from build123d import *

# Parameters (mm, degrees)
SKETCH1_R           = 12.5
BOSS_EXTRUDE1_DEPTH = 8
SKETCH2_R           = 10
BOSS_EXTRUDE2_DEPTH = 2
CUT_EXTRUDE1_REACH  = 22.31
SKETCH3_R           = 1.75
SKETCH4_R           = 3
CUT_EXTRUDE2_DEPTH  = 5
SKETCH5_R           = 9
SKETCH5_R_2         = 8
BOSS_EXTRUDE3_DEPTH = 1.5
CHAMFER1_SIZE       = 0.5


with BuildPart() as part:
    # Sketch1 → Boss-Extrude1 (new body)
    with BuildSketch(Plane(origin=(0, 0, 0), x_dir=(1, 0, 0), z_dir=(0, 1, 0))):
        with Locations(Location((0, 0, 0), (0, 0, 270))):
            Circle(SKETCH1_R)
    extrude(amount=BOSS_EXTRUDE1_DEPTH)

    # Sketch2 → Boss-Extrude2 (add)
    with BuildSketch(Plane(origin=(0, 8, 0), x_dir=(1, 0, 0), z_dir=(0, 1, 0))):
        with Locations(Location((0, 0, 0), (0, 0, 270))):
            Circle(SKETCH2_R)
    extrude(amount=BOSS_EXTRUDE2_DEPTH)

    # Sketch3 → Cut-Extrude1 (cut, up to next)
    with BuildSketch(Plane(origin=(0, 10, 0), x_dir=(1, 0, 0), z_dir=(0, 1, 0)), mode=Mode.PRIVATE) as cut_extrude1_sk1:
        with Locations(Location((0, 0, 0), (0, 0, 270))):
            Circle(SKETCH3_R)
    cut_extrude1_tool1 = extrude(cut_extrude1_sk1.sketch, amount=-CUT_EXTRUDE1_REACH, mode=Mode.PRIVATE) & part.part
    add(cut_extrude1_tool1.solids().sort_by_distance((0, 10, 0))[0], mode=Mode.SUBTRACT)

    # Sketch4 → Cut-Extrude2 (cut)
    with BuildSketch(Plane.XZ):
        with Locations(Location((0, 0, 0), (0, 0, 270))):
            Circle(SKETCH4_R)
    extrude(amount=-CUT_EXTRUDE2_DEPTH, mode=Mode.SUBTRACT)

    # Sketch5 → Boss-Extrude3 (add)
    with BuildSketch(Plane.XZ):
        with Locations(Location((0, 0, 0), (0, 0, 90))):
            Circle(SKETCH5_R)
        with Locations(Location((0, 0, 0), (0, 0, 270))):
            Circle(SKETCH5_R_2, mode=Mode.SUBTRACT)
    extrude(amount=BOSS_EXTRUDE3_DEPTH)

    # Chamfer1
    chamfer1_edges = [part.edges().sort_by_distance(p)[0] for p in [
        (0, 0, -12.5),
        (0, 8, -12.5),
    ]]
    chamfer(chamfer1_edges, length=CHAMFER1_SIZE)


solid = part.part
Design review of the part built by this model. Coordinates are the model's own, in mm. A direction names the side the tool comes from. Coordinates: 2 decimals unless noted, no trailing zeros. Loops run counter-clockwise (first coordinate to the right, second up) from the corner with the lowest first, then second, coordinate; pieces in that order, holes last.
Item 1: Add section A-A (z = 0). Write out the cut boundary in (x, y).
Completed:
outline: (-12.5, 0.5) - (-12, 0) - (-9, 0) - (-9, -1.5) - (-8, -1.5) - (-8, 0) - (-3, 0) - (-3, 5) - (-1.75, 5) - (-1.75, 10) - (-10, 10) - (-10, 8) - (-12, 8) - (-12.5, 7.5) - close; (1.75, 5) - (3, 5) - (3, 0) - (8, 0) - (8, -1.5) - (9, -1.5) - (9, 0) - (12, 0) - (12.5, 0.5) - (12.5, 7.5) - (12, 8) - (10, 8) - (10, 10) - (1.75, 10) - close
Item 2: Clearance check with flat-ended pins moving along their axes: pin 1 (2 mm diameter, centred on x = 9, y = 4, fed in from +Z); pin 2 (2 mm diameter, centred on x = 9.5, z = -7.5, fed in from +Y); pin 3 (5 mm diameter, centred on x = 1, z = 1, fed in from -Y). State where each tip first meets the part, or that it passes through.
Completed:
pin 1: stops at z = 9.6
pin 2: stops at y = 8
pin 3: stops at y = 0
Item 3: For faces 5 (the flat face through (9, 8, -5)), 6 (the flat face through (-2, 5, 0)), 7 (the cylindrical face through (-1.71, 7.54, -0.38)), list the 3-axis set-ups (+Z, -Z, +X, -X, +Y, -Y) from which the entire face can be reached by the end or side of a thin tool; tool diameter is ignored.
Completed:
face 5: +Y
face 6: -Y
face 7: +Y, -Y
Item 4: Draft analysis for pull direction X (two halves, no side actions). For faces 1 (the cylindrical face through (-2.703, -0.74, 8.584)), 2 (the flat face through (0.1, 0, 3.4)), 3 (the flat face through (0, 10, 2)), 4 (the cylindrical face through (0.9, 2.46, -2.86)), state which applies: pulls with the +X half, pulls with the -X half, needs draft (parallel to the pull), parting line crosses it, or undercut.
Completed:
face 1: parting line crosses it
face 2: undercut
face 3: needs draft
face 4: undercut
Item 5: Add section B-B (x = 0). Write out the cut boundary in (y, z).
Completed:
outline: (-1.5, -9) - (0, -9) - (0, -12) - (0.5, -12.5) - (7.5, -12.5) - (8, -12) - (8, -10) - (10, -10) - (10, -1.75) - (5, -1.75) - (5, -3) - (0, -3) - (0, -8) - (-1.5, -8) - close; (-1.5, 8) - (0, 8) - (0, 3) - (5, 3) - (5, 1.75) - (10, 1.75) - (10, 10) - (8, 10) - (8, 12) - (7.5, 12.5) - (0.5, 12.5) - (0, 12) - (0, 9) - (-1.5, 9) - close
Item 6: Add section D-D (y = 5.75). Write out the cut boundary in (x, z), and give its area (3 significant figures).
Completed:
outline: circle Ø25 at (0, 0); hole circle Ø3.5 at (0, 0)
area: 481 mm2
Item 7: Add section C-C (y = 3.5). Write out the cut boundary in (x, z).
Completed:
outline: circle Ø25 at (0, 0); hole circle Ø6 at (0, 0)
Item 8: Wall thickness on L1, parallel to X at y = -0.6, z = 0; L2, parallel to X at y = 8.1, z = 0; L3, parallel to Y at x = -4.5, z = 6: over which ranges is each line inside the solid? List them lowest first.
Completed:
L1: x = -9 to -8, 8 to 9
L2: x = -10 to -1.75, 1.75 to 10
L3: y = 0 to 10
